Read the model definition and answer for the solid it produces. Units are mm, in the model's axes. A direction names the side the tool comes from. Coordinates: 2 decimals unless noted, no trailing zeros. Write each loop counter-clockwise with the first axis right and the second up, starting at its lowest first coordinate (ties: lowest second). Pieces come first, ordered by that corner, then holes. Notation, with made-up numbers: M 84,31.5 L 140,31.5 A26 cw 140,67.5 Z; hole C 11,57 d10. An arc over 180 degrees is marked long. Use a Markdown table: item, result. Add a question column.
from build123d import *

# Parameters (mm, degrees)
F0_W     = 119.1
F0_H     = 82
F1_DEPTH = 5
F3_DEPTH = 63.1
F4_W     = 6.8
F4_H     = 2.5
F4_W_2   = 7
F4_W_3   = 6.5
F5_DEPTH = 53.3
F6_W     = 48
F6_H     = 2.5
F7_DEPTH = 27.8
F8_W     = 0.5
F8_H     = 70
F9_DEPTH = 25
F10_R    = 2
F11_R    = 0.5
F12_R    = 0.1


with BuildPart() as f1:
    # F0 (on Top) → F1 (new body)
    with BuildSketch(Plane.XY):
        with Locations((59.55, 41)):
            Rectangle(F0_W, F0_H)
    extrude(amount=F1_DEPTH)

    # F2 (on face) → F3 (cut)
    with BuildSketch(Plane.XY.offset(5)):
        Polygon((64.6, 76), (64.6, 25), (64.6, 6), (65.1, 6), (65.1, 76), align=None)
    extrude(amount=-F3_DEPTH, mode=Mode.SUBTRACT)

    # F4 (on face) → F5 (cut)
    with BuildSketch(Plane.XY.offset(5)):
        with Locations((32.3, 51.4)):
            Rectangle(F4_W, F4_H)
        Polygon((35.7, 50.15), (38.9217214942, 50.15), (41.1, 50.15), (41.1, 52.65), (35.7, 52.65), align=None)
        with Locations((44.6, 51.4)):
            Rectangle(F4_W_2, F4_H)
        with Locations((51.35, 51.4)):
            Rectangle(F4_W_3, F4_H)
        with Locations((19, 51.4)):
            Rectangle(F4_W, F4_H)
        with Locations((25.65, 51.4)):
            Rectangle(F4_W_3, F4_H)
        with Locations((58.1, 51.4)):
            Rectangle(F4_W_2, F4_H)
        with Locations((44.6, 30.6)):
            Rectangle(F4_W_2, F4_H)
        with Locations((32.3, 30.6)):
            Rectangle(F4_W, F4_H)
        with Locations((58.1, 30.6)):
            Rectangle(F4_W_2, F4_H)
        Polygon((41.1, 31.85), (38.9217214942, 31.85), (35.7, 31.85), (35.7, 29.35), (38, 29.35), (41.1, 29.35), align=None)
        with Locations((51.35, 30.6)):
            Rectangle(F4_W_3, F4_H)
        with Locations((25.65, 30.6)):
            Rectangle(F4_W_3, F4_H)
        with Locations((19, 30.6)):
            Rectangle(F4_W, F4_H)
    extrude(amount=-F5_DEPTH, mode=Mode.SUBTRACT)

    # F6 (on face) → F7 (cut)
    with BuildSketch(Plane.XY.offset(5)):
        with Locations((92.1, 51.4)):
            Rectangle(F6_W, F6_H)
        with Locations((92.1, 30.6)):
            Rectangle(F6_W, F6_H)
    extrude(amount=-F7_DEPTH, mode=Mode.SUBTRACT)

    # F8 (on face) → F9 (cut)
    with BuildSketch(Plane.XY.offset(5)):
        with Locations((9.25, 41)):
            Rectangle(F8_W, F8_H)
    extrude(amount=-F9_DEPTH, mode=Mode.SUBTRACT)

    # F10
    f10_edges = [f1.edges().sort_by_distance(p)[0] for p in [
        (119.1, 0, 2.5),
        (0, 0, 2.5),
        (119.1, 82, 2.5),
        (0, 82, 2.5),
    ]]
    fillet(f10_edges, radius=F10_R)

    # F11
    f11_edges = [f1.edges().sort_by_distance(p)[0] for p in [
        (15.6, 52.65, 2.5),
        (15.6, 50.15, 2.5),
        (61.6, 52.65, 2.5),
        (61.6, 50.15, 2.5),
        (68.1, 52.65, 2.5),
        (68.1, 50.15, 2.5),
        (116.1, 52.65, 2.5),
        (116.1, 50.15, 2.5),
        (116.1, 29.35, 2.5),
        (116.1, 31.85, 2.5),
        (68.1, 31.85, 2.5),
        (68.1, 29.35, 2.5),
        (15.6, 29.35, 2.5),
        (15.6, 31.85, 2.5),
        (61.6, 29.35, 2.5),
        (61.6, 31.85, 2.5),
    ]]
    fillet(f11_edges, radius=F11_R)

    # F12
    f12_edges = [f1.edges().sort_by_distance(p)[0] for p in [
        (64.6, 6, 2.5),
        (65.1, 6, 2.5),
        (64.6, 76, 2.5),
        (65.1, 76, 2.5),
        (9.5, 76, 2.5),
        (9, 76, 2.5),
        (9, 6, 2.5),
        (9.5, 6, 2.5),
    ]]
    fillet(f12_edges, radius=F12_R)


solid = f1.part
Item 1: Find section B-B on z = 4.25. Count the separate pieces of the cut face and the enclosed holes in it, then the cut area to 3 significant figures.
Item 2: Determine the mould class of faces 1 (the flat face through (9.5, 41, 3)), 2 (the flat face through (119.1, 40, 2)), 3 (the flat face through (59, 82, 2)), 4 (the flat face through (0, 40, 2)) for opening direction X: pulls with the +X half, pulls with the -X half, needs draft (parallel to the pull), parting line crosses it, or undercut.
Item 3: Find section A-A on x = 98.5. Give the vertices of the cut face in (y, z), then the cut area to 3 significant figures.
Item 4: For faces 5 (the flat face through (59, 42, 5)), 6 (the flat face through (92, 52.65, 3)), determine the directions among +Z, -Z, +X, -X, +Y, -Y from which every point of the face is accessible in a straight line to the end or side of a thin tool.
Item 5: Consider probe 1 along Y at (x, z) = (84.5, 4.15); probe 2 along X at (y, z) = (70, 3.6); probe 3 along X at (y, z) = (50.5, 0.6). Determine where each line is inside the solid, lowest interval first.
Geometry says:
| question | item | result |
|---|---|---|
| 1 | separate pieces | 1 |
| 1 | enclosed holes | 6 |
| 1 | area | 9,220 mm2 |
| 2 | face 1 | undercut |
| 2 | face 2 | pulls with the +X half |
| 2 | face 3 | needs draft |
| 2 | face 4 | pulls with the -X half |
| 3 | outline | M 0,0 L 29.35,0 L 29.35,5 L 0,5 Z; M 31.85,0 L 50.15,0 L 50.15,5 L 31.85,5 Z; M 52.65,0 L 82,0 L 82,5 L 52.65,5 Z |
| 3 | area | 385 mm2 |
| 4 | face 5 | +Z, +X, -X, +Y, -Y |
| 4 | face 6 | +Z, -Z |
| 5 | probe 1 | y = 0 to 29.35, 31.85 to 50.15, 52.65 to 82 |
| 5 | probe 2 | x = 0 to 9, 9.5 to 64.6, 65.1 to 119.1 |
| 5 | probe 3 | x = 0 to 9, 9.5 to 15.62, 61.58 to 64.6, 65.1 to 68.12, 116.08 to 119.1 |
